```python
from build123d import *

# Parameters (mm, degrees)
CROQUIS1_R              = 9
SALIENTE_EXTRUIR1_DEPTH = 53
CROQUIS2_R              = 8
SALIENTE_EXTRUIR2_DEPTH = 11.5
CROQUIS3_R              = 8.5
SALIENTE_EXTRUIR3_DEPTH = 2
SALIENTE_EXTRUIR4_DEPTH = 8
REDONDEO1_R             = 1
REDONDEO2_R             = 1


with BuildPart() as part:
    # Croquis1 → Saliente-Extruir1 (new body)
    with BuildSketch(Plane(origin=(0, 0, 0), x_dir=(1, 0, 0), z_dir=(0, 1, 0))):
        with Locations(Location((0, 0, 0), (0, 0, 270))):
            Circle(CROQUIS1_R)
    extrude(amount=SALIENTE_EXTRUIR1_DEPTH)

    # Croquis2 → Saliente-Extruir2 (add)
    with BuildSketch(Plane(origin=(0, 53, 0), x_dir=(1, 0, 0), z_dir=(0, 1, 0))):
        with Locations(Location((0, 0, 0), (0, 0, 270))):
            Circle(CROQUIS2_R)
    extrude(amount=SALIENTE_EXTRUIR2_DEPTH)

    # Croquis3 → Saliente-Extruir3 (add)
    with BuildSketch(Plane(origin=(0, 64.5, 0), x_dir=(1, 0, 0), z_dir=(0, 1, 0))):
        with Locations(Location((0, 0, 0), (0, 0, 270))):
            Circle(CROQUIS3_R)
    extrude(amount=SALIENTE_EXTRUIR3_DEPTH)

    # Croquis4 → Saliente-Extruir4 (add)
    with BuildSketch(Plane(origin=(0, 66.5, 0), x_dir=(1, 0, 0), z_dir=(0, 1, 0))):
        with BuildLine():
            Line((-3.3, -7.287660804), (-3.3, 2))
            Line((-3.3, 2), (3.3, 2))
            Line((3.3, 2), (3.3, -7.287660804))
            ThreePointArc((3.3, -7.287660804), (0, -8), (-3.3, -7.287660804))
        make_face()
    extrude(amount=SALIENTE_EXTRUIR4_DEPTH)

    # Redondeo1
    # the kernel refuses this fillet: 1 mm, written as the material it adds along each edge
    with BuildSketch(Plane(origin=(0, 66.5, 0), x_dir=(0.6410468977600248, 0, 0.7675017100125893), z_dir=(0.7675017100125893, 0, -0.6410468977600248))) as redondeo1_piece_1_section:
        with BuildLine():
            CenterArc((9, -0.866025404), REDONDEO1_R, 120, 60)
            Line((8, -0.866025404), (7.98, -0.866025404))
            Line((7.98, -0.866025404), (7.98, 0))
            Line((7.98, 0), (8, 0.02))
            ThreePointArc((8, 0.02), (8.25, 0.02), (8.49, 0.017320508))
            Line((8.49, 0.017320508), (8.5, 0))
        make_face()
    redondeo1_piece_1 = revolve(axis=Axis((0, 66.5, 0), (0, -1, 0)), revolution_arc=79.739856792, mode=Mode.PRIVATE)
    redondeo1_piece_1 = split(redondeo1_piece_1, bisect_by=Plane(origin=(3.3, 66.860958569, 8.125198581), z_dir=(-1, 0, 0)), keep=Keep.TOP, mode=Mode.PRIVATE)
    redondeo1_piece_1 = split(redondeo1_piece_1, bisect_by=Plane(origin=(-3.3, 66.860958569, 8.125198581), z_dir=(1, 0, 0)), keep=Keep.TOP, mode=Mode.PRIVATE)
    add(redondeo1_piece_1)
    with BuildSketch(Plane(origin=(3.3, 66.5, -2), x_dir=(1, 0, 0), z_dir=(0, 0, 1))) as redondeo1_piece_2_section:
        with BuildLine():
            CenterArc((REDONDEO1_R, REDONDEO1_R), REDONDEO1_R, 180, 90)
            Line((0, REDONDEO1_R), (-REDONDEO1_R * 0.02, REDONDEO1_R))
            Line((-REDONDEO1_R * 0.02, REDONDEO1_R), (-REDONDEO1_R * 0.02, -REDONDEO1_R * 0.02))
            Line((-REDONDEO1_R * 0.02, -REDONDEO1_R * 0.02), (REDONDEO1_R, -REDONDEO1_R * 0.02))
            Line((REDONDEO1_R, -REDONDEO1_R * 0.02), (REDONDEO1_R, 0))
        make_face()
    redondeo1_piece_2 = extrude(amount=11.787660804, mode=Mode.PRIVATE)
    redondeo1_piece_2 = redondeo1_piece_2 & Plane(origin=(0, 66.727902146, 0), x_dir=(0.4124999999999996, 0, 0.9109576005501028), z_dir=(0, -1, 0)) * Cylinder(8, 28, mode=Mode.PRIVATE)
    add(redondeo1_piece_2)
    with BuildSketch(Plane(origin=(-3.3, 66.5, -2), x_dir=(0, 0, -1), z_dir=(1, 0, 0))) as redondeo1_piece_3:
        with BuildLine():
            CenterArc((REDONDEO1_R, REDONDEO1_R), REDONDEO1_R, 180, 90)
            Line((0, REDONDEO1_R), (-REDONDEO1_R * 0.02, REDONDEO1_R))
            Line((-REDONDEO1_R * 0.02, REDONDEO1_R), (-REDONDEO1_R * 0.02, -REDONDEO1_R * 0.02))
            Line((-REDONDEO1_R * 0.02, -REDONDEO1_R * 0.02), (REDONDEO1_R, -REDONDEO1_R * 0.02))
            Line((REDONDEO1_R, -REDONDEO1_R * 0.02), (REDONDEO1_R, 0))
        make_face()
    extrude(amount=6.6)
    with BuildSketch(Plane(origin=(-3.3, 66.5, 9.787660804), x_dir=(-1, 0, 0), z_dir=(0, 0, -1))) as redondeo1_piece_4_section:
        with BuildLine():
            CenterArc((REDONDEO1_R, REDONDEO1_R), REDONDEO1_R, 180, 90)
            Line((0, REDONDEO1_R), (-REDONDEO1_R * 0.02, REDONDEO1_R))
            Line((-REDONDEO1_R * 0.02, REDONDEO1_R), (-REDONDEO1_R * 0.02, -REDONDEO1_R * 0.02))
            Line((-REDONDEO1_R * 0.02, -REDONDEO1_R * 0.02), (REDONDEO1_R, -REDONDEO1_R * 0.02))
            Line((REDONDEO1_R, -REDONDEO1_R * 0.02), (REDONDEO1_R, 0))
        make_face()
    redondeo1_piece_4 = extrude(amount=11.787660804, mode=Mode.PRIVATE)
    redondeo1_piece_4 = redondeo1_piece_4 & Plane(origin=(0, 66.727902035, 0), x_dir=(0.4124999999999996, 0, 0.9109576005501028), z_dir=(0, -1, 0)) * Cylinder(8, 28, mode=Mode.PRIVATE)
    add(redondeo1_piece_4)
    with BuildSketch(Plane(origin=(0, 66.5, 0), x_dir=(0.6410468977600248, 0, 0.7675017100125893), z_dir=(0.7675017100125893, 0, -0.6410468977600248))) as redondeo1_piece_5a_section:
        with BuildLine():
            CenterArc((9, -0.866025404), REDONDEO1_R, 120, 60)
            Line((8, -0.866025404), (7.98, -0.866025404))
            Line((7.98, -0.866025404), (7.98, 0))
            Line((7.98, 0), (8, 0.02))
            ThreePointArc((8, 0.02), (8.25, 0.02), (8.49, 0.017320508))
            Line((8.49, 0.017320508), (8.5, 0))
        make_face()
    redondeo1_piece_5a = revolve(axis=Axis((0, 66.5, 0), (0, -1, 0)), revolution_arc=79.739856792, mode=Mode.PRIVATE)
    redondeo1_piece_5a = split(redondeo1_piece_5a, bisect_by=Plane(origin=(3.3, 66.711912265, 6.883204996), z_dir=(1, 0, 0)), keep=Keep.TOP, mode=Mode.PRIVATE)
    with BuildSketch(Plane(origin=(3.3, 66.5, -2), x_dir=(1, 0, 0), z_dir=(0, 0, 1))) as redondeo1_piece_5b_section:
        with BuildLine():
            CenterArc((REDONDEO1_R, REDONDEO1_R), REDONDEO1_R, 180, 90)
            Line((0, REDONDEO1_R), (-REDONDEO1_R * 0.02, REDONDEO1_R))
            Line((-REDONDEO1_R * 0.02, REDONDEO1_R), (-REDONDEO1_R * 0.02, -REDONDEO1_R * 0.02))
            Line((-REDONDEO1_R * 0.02, -REDONDEO1_R * 0.02), (REDONDEO1_R, -REDONDEO1_R * 0.02))
            Line((REDONDEO1_R, -REDONDEO1_R * 0.02), (REDONDEO1_R, 0))
        make_face()
    redondeo1_piece_5b = extrude(amount=11.787660804, mode=Mode.PRIVATE)
    redondeo1_piece_5b = redondeo1_piece_5b & Plane(origin=(0, 66.724587575, 0), x_dir=(0, 0, 1), z_dir=(0, -1, 0)) * Cylinder(8.5, 28, mode=Mode.PRIVATE)
    redondeo1_piece_5b = redondeo1_piece_5b - Plane(origin=(0, 66.724587575, 0), x_dir=(0.4124999999999996, 0, 0.9109576005501028), z_dir=(0, -1, 0)) * Cylinder(8, 28, mode=Mode.PRIVATE)
    redondeo1_piece_5 = redondeo1_piece_5a & redondeo1_piece_5b
    add(redondeo1_piece_5)
    with BuildSketch(Plane(origin=(0, 66.5, 0), x_dir=(0.6410468977600248, 0, 0.7675017100125893), z_dir=(0.7675017100125893, 0, -0.6410468977600248))) as redondeo1_piece_6a_section:
        with BuildLine():
            CenterArc((9, -0.866025404), REDONDEO1_R, 120, 60)
            Line((8, -0.866025404), (7.98, -0.866025404))
            Line((7.98, -0.866025404), (7.98, 0))
            Line((7.98, 0), (8, 0.02))
            ThreePointArc((8, 0.02), (8.25, 0.02), (8.49, 0.017320508))
            Line((8.49, 0.017320508), (8.5, 0))
        make_face()
    redondeo1_piece_6a = revolve(axis=Axis((0, 66.5, 0), (0, -1, 0)), revolution_arc=79.739856792, mode=Mode.PRIVATE)
    redondeo1_piece_6a = split(redondeo1_piece_6a, bisect_by=Plane(origin=(-3.3, 66.71191226, 6.883204989), z_dir=(-1, 0, 0)), keep=Keep.TOP, mode=Mode.PRIVATE)
    with BuildSketch(Plane(origin=(-3.3, 66.5, 9.787660804), x_dir=(-1, 0, 0), z_dir=(0, 0, -1))) as redondeo1_piece_6b_section:
        with BuildLine():
            CenterArc((REDONDEO1_R, REDONDEO1_R), REDONDEO1_R, 180, 90)
            Line((0, REDONDEO1_R), (-REDONDEO1_R * 0.02, REDONDEO1_R))
            Line((-REDONDEO1_R * 0.02, REDONDEO1_R), (-REDONDEO1_R * 0.02, -REDONDEO1_R * 0.02))
            Line((-REDONDEO1_R * 0.02, -REDONDEO1_R * 0.02), (REDONDEO1_R, -REDONDEO1_R * 0.02))
            Line((REDONDEO1_R, -REDONDEO1_R * 0.02), (REDONDEO1_R, 0))
        make_face()
    redondeo1_piece_6b = extrude(amount=11.787660804, mode=Mode.PRIVATE)
    redondeo1_piece_6b = redondeo1_piece_6b & Plane(origin=(0, 66.72458755, 0), x_dir=(0, 0, 1), z_dir=(0, -1, 0)) * Cylinder(8.5, 28, mode=Mode.PRIVATE)
    redondeo1_piece_6b = redondeo1_piece_6b - Plane(origin=(0, 66.72458755, 0), x_dir=(0.4124999999999996, 0, 0.9109576005501028), z_dir=(0, -1, 0)) * Cylinder(8, 28, mode=Mode.PRIVATE)
    redondeo1_piece_6 = redondeo1_piece_6a & redondeo1_piece_6b
    add(redondeo1_piece_6)
    with BuildSketch(Plane(origin=(3.3, 66.5, -4.5), x_dir=(1, 0, 0), z_dir=(0, 0, 1))) as redondeo1_piece_7a_section:
        with BuildLine():
            CenterArc((REDONDEO1_R, REDONDEO1_R), REDONDEO1_R, 180, 90)
            Line((0, REDONDEO1_R), (-REDONDEO1_R * 0.02, REDONDEO1_R))
            Line((-REDONDEO1_R * 0.02, REDONDEO1_R), (-REDONDEO1_R * 0.02, -REDONDEO1_R * 0.02))
            Line((-REDONDEO1_R * 0.02, -REDONDEO1_R * 0.02), (REDONDEO1_R, -REDONDEO1_R * 0.02))
            Line((REDONDEO1_R, -REDONDEO1_R * 0.02), (REDONDEO1_R, 0))
        make_face()
    redondeo1_piece_7a = extrude(amount=14.287660804, mode=Mode.PRIVATE)
    redondeo1_piece_7a = split(redondeo1_piece_7a, bisect_by=Plane(origin=(3.526395114, 66.726395114, -2), z_dir=(0, 0, -1)), keep=Keep.TOP, mode=Mode.PRIVATE)
    with BuildSketch(Plane(origin=(-3.3, 66.5, -2), x_dir=(0, 0, -1), z_dir=(1, 0, 0))) as redondeo1_piece_7b_section:
        with BuildLine():
            CenterArc((REDONDEO1_R, REDONDEO1_R), REDONDEO1_R, 180, 90)
            Line((0, REDONDEO1_R), (-REDONDEO1_R * 0.02, REDONDEO1_R))
            Line((-REDONDEO1_R * 0.02, REDONDEO1_R), (-REDONDEO1_R * 0.02, -REDONDEO1_R * 0.02))
            Line((-REDONDEO1_R * 0.02, -REDONDEO1_R * 0.02), (REDONDEO1_R, -REDONDEO1_R * 0.02))
            Line((REDONDEO1_R, -REDONDEO1_R * 0.02), (REDONDEO1_R, 0))
        make_face()
    redondeo1_piece_7b = extrude(amount=9.1, mode=Mode.PRIVATE)
    redondeo1_piece_7b = split(redondeo1_piece_7b, bisect_by=Plane(origin=(3.3, 66.726395114, -2.226395114), z_dir=(1, 0, 0)), keep=Keep.TOP, mode=Mode.PRIVATE)
    redondeo1_piece_7 = redondeo1_piece_7a & redondeo1_piece_7b
    add(redondeo1_piece_7)
    with BuildSketch(Plane(origin=(-5.8, 66.5, -2), x_dir=(0, 0, -1), z_dir=(1, 0, 0))) as redondeo1_piece_8a_section:
        with BuildLine():
            CenterArc((REDONDEO1_R, REDONDEO1_R), REDONDEO1_R, 180, 90)
            Line((0, REDONDEO1_R), (-REDONDEO1_R * 0.02, REDONDEO1_R))
            Line((-REDONDEO1_R * 0.02, REDONDEO1_R), (-REDONDEO1_R * 0.02, -REDONDEO1_R * 0.02))
            Line((-REDONDEO1_R * 0.02, -REDONDEO1_R * 0.02), (REDONDEO1_R, -REDONDEO1_R * 0.02))
            Line((REDONDEO1_R, -REDONDEO1_R * 0.02), (REDONDEO1_R, 0))
        make_face()
    redondeo1_piece_8a = extrude(amount=9.1, mode=Mode.PRIVATE)
    redondeo1_piece_8a = split(redondeo1_piece_8a, bisect_by=Plane(origin=(-3.3, 66.726395114, -2.226395114), z_dir=(-1, 0, 0)), keep=Keep.TOP, mode=Mode.PRIVATE)
    with BuildSketch(Plane(origin=(-3.3, 66.5, 9.787660804), x_dir=(-1, 0, 0), z_dir=(0, 0, -1))) as redondeo1_piece_8b_section:
        with BuildLine():
            CenterArc((REDONDEO1_R, REDONDEO1_R), REDONDEO1_R, 180, 90)
            Line((0, REDONDEO1_R), (-REDONDEO1_R * 0.02, REDONDEO1_R))
            Line((-REDONDEO1_R * 0.02, REDONDEO1_R), (-REDONDEO1_R * 0.02, -REDONDEO1_R * 0.02))
            Line((-REDONDEO1_R * 0.02, -REDONDEO1_R * 0.02), (REDONDEO1_R, -REDONDEO1_R * 0.02))
            Line((REDONDEO1_R, -REDONDEO1_R * 0.02), (REDONDEO1_R, 0))
        make_face()
    redondeo1_piece_8b = extrude(amount=14.287660804, mode=Mode.PRIVATE)
    redondeo1_piece_8b = split(redondeo1_piece_8b, bisect_by=Plane(origin=(-3.526395114, 66.726395114, -2), z_dir=(0, 0, -1)), keep=Keep.TOP, mode=Mode.PRIVATE)
    redondeo1_piece_8 = redondeo1_piece_8a & redondeo1_piece_8b
    add(redondeo1_piece_8)

    # Redondeo2
    redondeo2_edges = [part.edges().sort_by_distance(p)[0] for p in [
        (0, 74.5, 8),
        (3.3, 74.5, 2.643830402),
        (0, 74.5, -2),
        (-3.3, 74.5, 2.643830402),
    ]]
    fillet(redondeo2_edges, radius=REDONDEO2_R)


solid = part.part
```
The listing builds one solid part. Answer for the finished solid, in the listing's coordinates (mm). A direction names the side the tool comes from. Give positions to 0.01 mm unless a question says otherwise; leave off trailing zeros. Loops run counter-clockwise (first coordinate to the right, second up) from the corner with the lowest first, then second, coordinate; pieces in that order, holes last. Notation, with made-up numbers: (43.5, 77) - (85.5, 77) arc R16 cw to (85.5, 98) - close; hole circle Ø9 at (60, -13). An arc over 180 degrees is marked (long way). Return JSON: item names as keys, results as strings. Group by question number.
1. Find section C-C (y = 61.5). Write down the section's boundary in (x, z), then the cut area to 3 significant figures.
2. Find section D-D (x = -5.25). Write down the section's boundary in (y, z), then the cut area to 3 significant figures.
3. Which of the six approach directions +Z, -Z, +X, -X, +Y, -Y give full straight-line access (tool end or side, diameter ignored) to faces 1 (the flat face through (0, 71, -2)), 2 (the cylindrical face through (8.428, 65.486, -1.107)), 3 (the flat face through (-3.3, 71, 3))?
4. Determine the mould class of faces 4 (the flat face through (3.3, 70, 3)), 5 (the cylindrical face through (-7.81, 58.67, -1.73)), 6 (the flat face through (0, 66.5, -4)) for opening direction Y: pulls with the +Y half, pulls with the -Y half, needs draft (parallel to the pull), parting line crosses it, or undercut.
5. Given pin 1 Ø1.5 at (x, y) = (2, 36) entering from -Z; pin 2 Ø5 at (y, z) = (71.5, 1.5) entering from +X; pin 3 Ø3 at (x, y) = (0.5, 23.5) entering from -Z; pin 4 Ø5 at (x, y) = (0, 71.5) entering from -Z, each flat-ended and moving along its own axis, determine where each tip first touches the part or whether it passes through.
6. Find section B-B (z = 0). Write down the section's boundary in (x, y).
7. Straight lines are drawn through the part: line 1 (Y direction, x = -6.5, z = -3.75); line 2 (X direction, y = 59.5, z = 0.5); line 3 (Z direction, x = 1.5, y = 38). For each, find the intervals that lie inside material, in ascending order. Write a range as [from, to].
8. Find section A-A (x = 0). Write down the section's boundary in (y, z), then the cut area to 3 significant figures.
Verdict:
{
 "1": {"outline": "circle Ø16 at (0, 0)", "area": "201 mm^2"},
 "2": {"outline": "(0, -7.31) - (53, -7.31) - (53, -6.04) - (64.5, -6.04) - (64.5, -6.68) - (66.5, -6.68) - (66.5, 6.68) - (64.5, 6.68) - (64.5, 6.04) - (53, 6.04) - (53, 7.31) - (0, 7.31) - close", "area": "940 mm^2"},
 "3": {"face 1": "-Z, +X, -X, +Y", "face 2": "+Y", "face 3": "+Z, -Z, -X, +Y"},
 "4": {"face 4": "needs draft", "face 5": "undercut", "face 6": "pulls with the +Y half"},
 "5": {"pin 1": "stops at z = -8.91", "pin 2": "stops at x = 3.3", "pin 3": "stops at z = -9", "pin 4": "stops at z = -2"},
 "6": {"outline": "(-9, 0) - (9, 0) - (9, 53) - (8, 53) - (8, 64.5) - (8.5, 64.5) - (8.5, 66.5) - (4.3, 66.5) arc R1 cw to (3.3, 67.5) - (3.3, 73.5) arc R1 ccw to (2.3, 74.5) - (-2.3, 74.5) arc R1 ccw to (-3.3, 73.5) - (-3.3, 67.5) arc R1 cw to (-4.3, 66.5) - (-8.5, 66.5) - (-8.5, 64.5) - (-8, 64.5) - (-8, 53) - (-9, 53) - close"},
 "7": {"line 1": "y = [0, 66.5]", "line 2": "x = [-7.98, 7.98]", "line 3": "z = [-8.87, 8.87]"},
 "8": {"outline": "(0, -9) - (53, -9) - (53, -8) - (64.5, -8) - (64.5, -8.5) - (66.5, -8.5) - (66.5, -3) arc R1 cw to (67.5, -2) - (73.5, -2) arc R1 ccw to (74.5, -1) - (74.5, 7) arc R1 ccw to (73.5, 8) - (67.37, 8) arc R1 cw to (66.5, 8.5) - (64.5, 8.5) - (64.5, 8) - (53, 8) - (53, 9) - (0, 9) - close", "area": "1,250 mm^2"}
}
